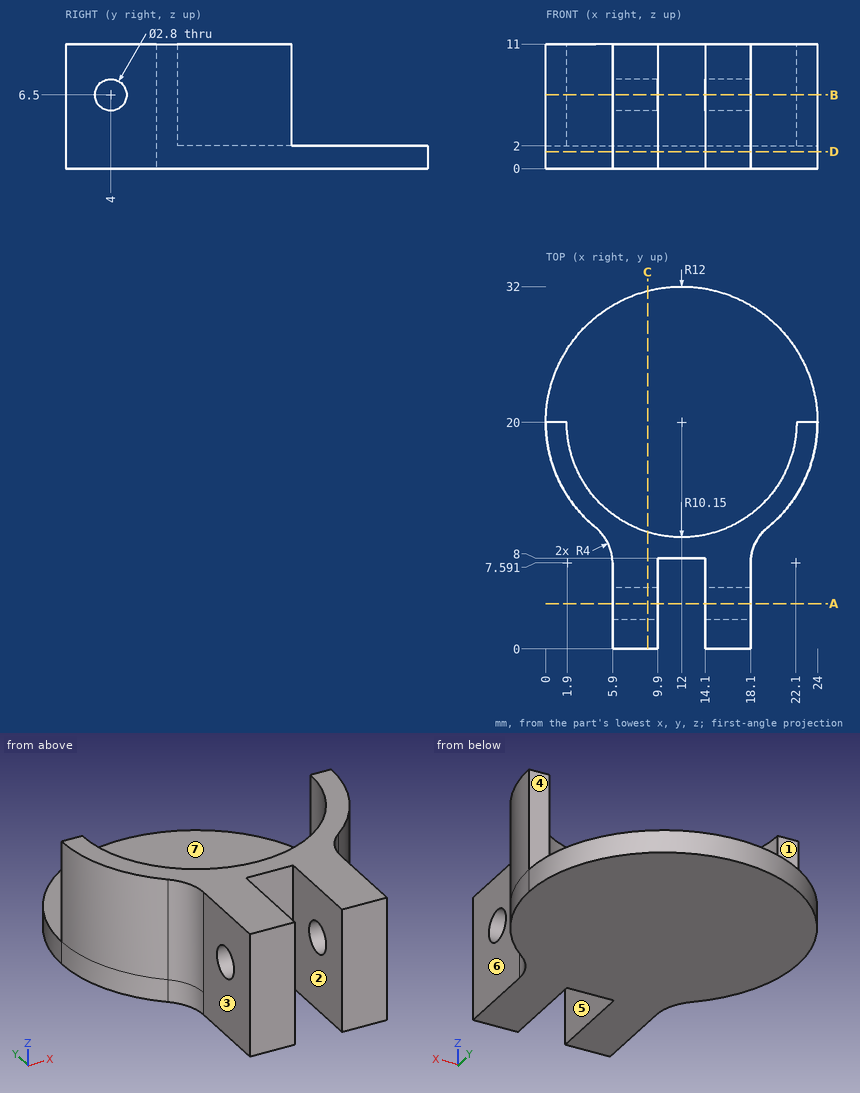
Print and shaded views of the part. All mm, measured from the part's lowest x, y and z. A direction names the side the tool comes from. Give positions to 0.01 mm unless a question says otherwise; leave off trailing zeros. Loops run counter-clockwise (first coordinate to the right, second up) from the corner with the lowest first, then second, coordinate; pieces in that order, holes last. Notation, with made-up numbers: (5, 75) - (15, 75) arc R33 ccw to (15, 113) - close; hole circle Ø1 at (0, -12). An arc over 180 degrees is marked (long way). Use a Markdown table: item, result.
(1) Which spindle directions (+Z, -Z, +X, -X, +Y, -Y) get a long thin tool onto all of the face, cutting with end or side? Do the marked faces 4, 5, 6 and 7. Say none if no direction does.
Taken from the geometry:
| item | result |
|---|---|
| face 4 | +Z, +X, -X, +Y |
| face 5 | +Z, -Z, -Y |
| face 6 | +Z, -Z, +X, -Y |
| face 7 | +Z, +Y |
(2) Band-saw the part on A-A (y = 4). Give the cut face in (x, z).
Taken from the geometry:
| item | result |
|---|---|
| outline | (5.9, 0) - (9.9, 0) - (9.9, 5.1) - (5.9, 5.1) - close; (5.9, 7.9) - (9.9, 7.9) - (9.9, 11) - (5.9, 11) - close; (14.1, 0) - (18.1, 0) - (18.1, 5.1) - (14.1, 5.1) - close; (14.1, 7.9) - (18.1, 7.9) - (18.1, 11) - (14.1, 11) - close |
(3) Drop flat-ended pins along their axis: pin 1 Ø3.5 at (x, z) = (13, 4.5) entering from -Y; pin 2 Ø2 at (x, y) = (7, 20) entering from +Z; pin 3 Ø2.5 at (y, z) = (2, 6) entering from -X; pin 4 Ø4 at (y, z) = (5, 3) entering from +X. Give the stop position or say it passes through.
Taken from the geometry:
| item | result |
|---|---|
| pin 1 | y = 0 |
| pin 2 | z = 2 |
| pin 3 | x = 5.9 |
| pin 4 | x = 18.1 |
(4) Band-saw the part on D-D (z = 1.5). Give the cut face in (x, y) (1 decimal), and give its area (3 significant figures).
Taken from the geometry:
| item | result |
|---|---|
| outline | (4.4, 10.7) arc R4 cw to (5.9, 7.6) - (5.9, 0) - (9.9, 0) - (9.9, 8) - (14.1, 8) - (14.1, 0) - (18.1, 0) - (18.1, 7.6) arc R4 cw to (19.6, 10.7) arc R12 ccw (long way) to start |
| area | 524 mm2 |
(5) Wall check: line 1 along Z through (x, y) = (6.75, 4); line 2 along X through (y, z) = (6.5, 6.75); line 3 along Z through (x, y) = (7.75, 20.5). Give the ranges that are in metal, low to high.
Taken from the geometry:
| item | result |
|---|---|
| line 1 | 0 to 5.1, 7.9 to 11 |
| line 2 | 5.9 to 9.9, 14.1 to 18.1 |
| line 3 | 0 to 2 |
(6) Pull direction X, two halves, no side cores. Call the marked faces 1, 2 and 3: +X half, -X half, draft (parallel to the pull), parting line (faces both ways), or undercut.
Taken from the geometry:
| item | result |
|---|---|
| face 1 | draft |
| face 2 | undercut |
| face 3 | -X half |
(7) Band-saw the part on B-B (z = 6.5). Give the number of separate pieces and of enclosed holes in the cut face, and give its area (3 significant figures).
Taken from the geometry:
| item | result |
|---|---|
| separate pieces | 3 |
| enclosed holes | 0 |
| area | 114 mm2 |
(8) Band-saw the part on C-C (x = 9). Give the cut face in (y, z), and give its area (3 significant figures).
Taken from the geometry:
| item | result |
|---|---|
| outline | (0, 0) - (31.62, 0) - (31.62, 2) - (10.3, 2) - (10.3, 11) - (0, 11) - close; hole circle Ø2.8 at (4, 6.5) |
| area | 150 mm2 |
